For this review, take the finished solid that the model builds, in its own axes (mm). Face numbers are marked on the shaded views. A direction names the side the tool comes from. Round coordinates to 2 decimals unless told otherwise and drop trailing zeros. Loops run counter-clockwise (first coordinate to the right, second up) from the corner with the lowest first, then second, coordinate; pieces in that order, holes last. Notation, with made-up numbers: M -8.75,25.5 L 48.25,25.5 A7 cw 48.25,29.5 Z; hole C 62,76.25 d8. An arc over 180 degrees is marked long. One line per question, with ' | ' between items. Start each with the question number.
1) Mouldability with a two-part tool opening along X and no side actions: class the marked faces 1, 2, 3 and 4 as pulls with the +X half, pulls with the -X half, needs draft (parallel to the pull), parting line crosses it, or undercut.
2) We need section B-B (y = 15.5). Give the boundary of the cut face in (x, z), and give its area (4 significant figures).
3) We need section D-D (y = -7). Give the boundary of the cut face in (x, z).
4) For pin 1 Ø1.9 at (x, y) = (-13.5, -26) entering from -Z; pin 2 Ø1 at (x, y) = (12.5, 0) entering from -Z; pin 3 Ø2.5 at (x, y) = (-13.5, 25.5) entering from +Z; pin 4 Ø1 at (x, z) = (11, 2) entering from +Y, all flat-tipped, find the tip position at first contact; note any pin that passes through.
5) We need section C-C (x = 7). Give the boundary of the cut face in (y, z).
6) We need section A-A (y = 35.5). Give the boundary of the cut face in (x, z).
7) For probe 1 along X at (y, z) = (-26, 1.3); probe 2 along Y at (x, z) = (15, 3.2); probe 3 along X at (y, z) = (26, 1.4), list the stretches that pass through material, from the lowest coordinate up. Write a range as from..to.
8) For the marked faces 5 and 6, list the 3-axis set-ups (+Z, -Z, +X, -X, +Y, -Y) from which the entire face can be reached by the end or side of a thin tool; tool diameter is ignored.
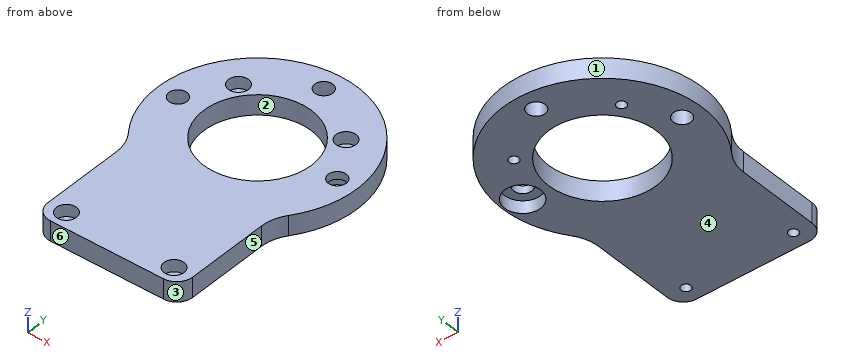
```python
from build123d import *

# Parameters (mm, degrees)
SKETCH_1_R                   = 1.2
SKETCH_1_R_2                 = 13.5
EXTRUDE_1_DEPTH              = 5
SKETCH_2_R                   = 2.5
CUT_EXTRUDE_1_DEPTH          = 3
SKETCH_3_R                   = 2.25
CUT_EXTRUDE_2_DEPTH          = 1
CUT_EXTRUDE_2_DEPTH_BACK     = 6
HOLE_WIZARD_M4_2_D           = 4.5
HOLE_WIZARD_M4_2_CBORE_D     = 9
HOLE_WIZARD_M4_2_CBORE_DEPTH = 3.1


with BuildPart() as part:
    # 스케치1 → 보스-돌출1 (new body)
    with BuildSketch(Plane.XY):
        with BuildLine():
            Line((18.188636287, -5.246102869), (18.188636287, -26))
            ThreePointArc((18.188636287, -26), (17.017063412, -28.828427125), (14.188636287, -30))
            Line((14.188636287, -30), (-14.188636287, -30))
            ThreePointArc((-14.188636287, -30), (-17.017063412, -28.828427125), (-18.188636287, -26))
            Line((-18.188636287, -26), (-18.188636287, -5.246102869))
            ThreePointArc((-18.188636287, -5.246102869), (-18.687611058, -2.126724792), (-20.134740205, 0.681355093))
            ThreePointArc((-20.134740205, 0.681355093), (0, 40.5), (20.134740205, 0.681355093))
            ThreePointArc((20.134740205, 0.681355093), (18.687611058, -2.126724792), (18.188636287, -5.246102869))
        make_face()
        with Locations((-13.5, 26)):
            Circle(SKETCH_1_R, mode=Mode.SUBTRACT)
        with Locations((13.5, 26)):
            Circle(SKETCH_1_R, mode=Mode.SUBTRACT)
        with Locations((-13.5, -26)):
            Circle(SKETCH_1_R, mode=Mode.SUBTRACT)
        with Locations((13.5, -26)):
            Circle(SKETCH_1_R, mode=Mode.SUBTRACT)
        with Locations((0, 15.5)):
            Circle(SKETCH_1_R_2, mode=Mode.SUBTRACT)
    extrude(amount=EXTRUDE_1_DEPTH)

    # 스케치2 → 컷-돌출1 (cut)
    with BuildSketch(Plane.XY.offset(5)):
        with Locations((-13.5, 26)):
            Circle(SKETCH_2_R)
        with Locations((13.5, 26)):
            Circle(SKETCH_2_R)
        with Locations((-13.5, -26)):
            Circle(SKETCH_2_R)
        with Locations((13.5, -26)):
            Circle(SKETCH_2_R)
    extrude(amount=-CUT_EXTRUDE_1_DEPTH, mode=Mode.SUBTRACT)

    # 스케치3 → 컷-돌출2 (cut, two sides)
    with BuildSketch(Plane.XY.offset(5)) as cut_extrude_2_sk:
        with Locations((-19.982848321, 15.5)):
            Circle(SKETCH_3_R)
        with Locations((0.017151679, 35.5)):
            Circle(SKETCH_3_R)
    extrude(amount=CUT_EXTRUDE_2_DEPTH, mode=Mode.SUBTRACT)
    extrude(cut_extrude_2_sk.sketch, amount=-CUT_EXTRUDE_2_DEPTH_BACK, mode=Mode.SUBTRACT)

    # M4 남비 머리 나사용 카운터보어2 (through all)
    with Locations(Plane(origin=(0, 0, 0), x_dir=(-1, 0, 0), z_dir=(0, 0, -1))):
        with Locations((-20.017151679, 15.5)):
            CounterBoreHole(HOLE_WIZARD_M4_2_D / 2, HOLE_WIZARD_M4_2_CBORE_D / 2, HOLE_WIZARD_M4_2_CBORE_DEPTH)


solid = part.part
```
Answers below:
1) face 1: parting line crosses it | face 2: undercut | face 3: pulls with the +X half | face 4: needs draft
2) outline: M -25,0 L -22.23,0 L -22.23,5 L -25,5 Z; M -17.73,0 L -13.5,0 L -13.5,5 L -17.73,5 Z; M 13.5,0 L 15.52,0 L 15.52,3.1 L 17.77,3.1 L 17.77,5 L 13.5,5 Z; M 22.27,3.1 L 24.52,3.1 L 24.52,0 L 25,0 L 25,5 L 22.27,5 Z | area: 56.05 mm^2
3) outline: M -18.19,0 L 18.19,0 L 18.19,5 L -18.19,5 Z
4) pin 1: through | pin 2: z = 0 | pin 3: z = 2 | pin 4: y = 38.19
5) outline: M -30,0 L 3.96,0 L 3.96,5 L -30,5 Z; M 27.04,0 L 39.5,0 L 39.5,5 L 27.04,5 Z
6) outline: M -15,0 L -2.23,0 L -2.23,5 L -15,5 Z; M 2.27,0 L 15,0 L 15,5 L 2.27,5 Z
7) probe 1: -18.19..-14.7, -12.3..12.3, 14.7..18.19 | probe 2: -29.92..-28, -24..24, 28..35.5 | probe 3: -22.69..-14.7, -12.3..-8.49, 8.49..12.3, 14.7..22.69
8) face 5: +Z, -Z, +X, -Y | face 6: +Z, -Z, +X, -X, -Y
